Could you check a few things on this model? Use its own coordinates, in mm. A direction names the side the tool comes from. Give positions to 0.01 mm unless a question says otherwise; leave off trailing zeros. Write each loop counter-clockwise with the first axis right and the second up, starting at its lowest first coordinate (ties: lowest second). Pieces come first, ordered by that corner, then holes. Notation, with made-up numbers: (38, 87) -> (81, 87) arc R26 ccw to (81, 112) -> close; hole circle Ø7 at (-11, 63.5). An arc over 180 degrees is marked (long way). Write item = value, one per line. Start each with the question number.
```python
from build123d import *

# Parameters (mm, degrees)
SKETCH1_R           = 25
BOSS_EXTRUDE1_DEPTH = 8
SKETCH2_R           = 8.664977056
BOSS_EXTRUDE2_DEPTH = 50
SKETCH3_R           = 6
CUT_EXTRUDE1_DEPTH  = 15


with BuildPart() as part:
    # Sketch1 → Boss-Extrude1 (new body)
    with BuildSketch(Plane(origin=(0, 0, 0), x_dir=(1, 0, 0), z_dir=(0, 1, 0))):
        Circle(SKETCH1_R)
    extrude(amount=BOSS_EXTRUDE1_DEPTH)

    # Sketch2 → Boss-Extrude2 (add)
    with BuildSketch(Plane(origin=(0, 8, 0), x_dir=(1, 0, 0), z_dir=(0, 1, 0))):
        Circle(SKETCH2_R)
    extrude(amount=BOSS_EXTRUDE2_DEPTH)

    # Sketch3 → Cut-Extrude1 (cut)
    with BuildSketch(Plane(origin=(20, 0, 0), x_dir=(0, 0, -1), z_dir=(1, 0, 0))):
        with Locations((0, 29.42990961)):
            Circle(SKETCH3_R)
    extrude(amount=-CUT_EXTRUDE1_DEPTH, mode=Mode.SUBTRACT)


solid = part.part
```
(1) On a 3-axis mill with a long thin cutter (end or side, diameter ignored), from which of +Z, -Z, +X, -X, +Y, -Y can I reach the whole of each face in a straight line? I mean faces 5 (the flat face through (0, 8, 11)), 6 (the cylindrical face through (23.846, 3.944, -7.509)). Say none if no direction works.
(2) We'd pull the mould along Y, two halves only. Please class faces 1 (the cylindrical face through (6.45, 27.13, -5.54)), 2 (the flat face through (5, 30, 0)), 3 (the flat face through (0, 58, 0)), 4 (the flat face through (0, 0, 0)): released by +Y, released by -Y, zero draft, split by the parting line, or undercut.
(3) Imagine slicing it at A-A (x = 0). Please give me the cut outline in (y, z), then the cut area to 3 significant figures.
(4) Imagine slicing it at D-D (z = 7.5). Please give me the cut outline in (x, y), then the cut area to 3 significant figures.
(5) I'm going to push flat-ended pins straight in: pin 1 (8 mm diameter, centred on x = 16, y = 19.5, fed in from -Z); pin 2 (6 mm diameter, centred on y = 31.5, z = 2.5, fed in from +X); pin 3 (1 mm diameter, centred on y = 16, z = -5.5, fed in from +X); pin 4 (15.5 mm diameter, centred on y = 29.43, z = 0, fed in from +X) (3 decimals). Where does each tip first touch, or does it pass through?
(6) If I drill on line 1 along Y through (x, z) = (7.8, 0); line 2 along Y through (x, z) = (16.5, 15.5); line 3 along X through (y, z) = (50.5, -0.5), over which ranges is the centre line in solid material (lowest first)? Write a range as from..to.
(7) Imagine slicing it at B-B (z = 0). Please give me the cut outline in (x, y), then the cut area to 3 significant figures.
(8) Imagine slicing it at C-C (y = 46). Please give me the cut outline in (x, z).
Answers below:
q1.face_5 = +Y
q1.face_6 = +Y, -Y
q2.face_1 = undercut
q2.face_2 = undercut
q2.face_3 = released by +Y
q2.face_4 = released by -Y
q3.outline = (0, -25) -> (8, -25) -> (8, -8.66) -> (58, -8.66) -> (58, 8.66) -> (8, 8.66) -> (8, 25) -> (0, 25) -> close
q3.area = 1,270 mm^2
q4.outline = (-23.85, 0) -> (23.85, 0) -> (23.85, 8) -> (4.34, 8) -> (4.34, 58) -> (-4.34, 58) -> (-4.34, 8) -> (-23.85, 8) -> close
q4.area = 816 mm^2
q5.pin_1 = through
q5.pin_2 = 7.96
q5.pin_3 = 7.08
q5.pin_4 = 8.665
q6.line_1 = 0..23.43, 35.43..58
q6.line_2 = 0..8
q6.line_3 = -8.65..8.65
q7.outline = (-25, 0) -> (25, 0) -> (25, 8) -> (8.66, 8) -> (8.66, 23.43) -> (5, 23.43) -> (5, 35.43) -> (8.66, 35.43) -> (8.66, 58) -> (-8.66, 58) -> (-8.66, 8) -> (-25, 8) -> close
q7.area = 1,220 mm^2
q8.outline = circle Ø17.33 at (0, 0)
